Geometry: final body of the model. Coordinates: model frame, mm. A direction names the side the tool comes from. Give positions to 0.01 mm unless a question says otherwise; leave off trailing zeros. Loops run counter-clockwise (first coordinate to the right, second up) from the corner with the lowest first, then second, coordinate; pieces in that order, holes last. Notation, with made-up numbers: (12, 56) -> (69, 56) arc R30 ccw to (69, 82) -> close; hole circle Ø5 at (-33.5, 79.5). An arc over 180 degrees is marked (long way). Answer in a Markdown table with one row per item. Add a question column.
1) Section query C-C (y = 77). Return the cut outline in (x, z), plus the area to 3 significant figures.
2) Section query B-B (x = -15.5). Return the cut outline in (y, z), plus the area to 3 significant figures.
3) Section query D-D (x = 0). Return the cut outline in (y, z), plus the area to 3 significant figures.
4) First-contact query: P1, Ø5, axis at x = -22, z = 4.5, coming from the -Y side; P2, Ø8, axis at x = 16.5, z = 8.5, coming from the -Y side; P3, Ø5, axis at x = 20.5, z = -27, coming from the +Y side. Flat tips, straight axial feed; report the tip coordinate or a pass-through.
5) Section query A-A (z = 0). Return the cut outline in (x, y), plus the area to 3 significant figures.
6) Draft query along Y for faces 1 (the flat face through (-20, -40, 0)), 2 (the flat face through (-8, 0, -1)), 3 (the cylindrical face through (0.33, -9.844, 7.493)), 4 (the flat face through (-8, 5, -1)). Return one class per face: +Y half, -Y half, draft (parallel to the pull), parting line (faces both ways), or undercut.
7) Access query for faces 5 (the cylindrical face through (1.802, 69.09, 5.723)), 6 (the cylindrical face through (-0.28, -28.27, 0.65)), 7 (the flat face through (20, -40, 0)). Directions: +Z, -Z, +X, -X, +Y, -Y. A direction counts if a zero-diameter tool reaches every point of the face in a straight line with its end or side. Return the directions, or none.
8) Line query: line 1 (Y direction, x = 0, z = 0); line 2 (Y direction, x = -26, z = -5); line 3 (Z direction, x = -1, y = 4). Output: solid intervals per line, ascending. Write a range as from..to.
```python
from build123d import *

# Parameters (mm, degrees)
SKETCH4_R           = 39
BOSS_EXTRUDE2_DEPTH = 5
SKETCH5_R           = 6
BOSS_EXTRUDE3_DEPTH = 130
SKETCH6_R           = 7.5
BOSS_EXTRUDE4_DEPTH = 20
SKETCH8_R           = 15.233231967
SKETCH8_R_2         = 5
BOSS_EXTRUDE5_DEPTH = 20


with BuildPart() as part:
    # Sketch4 → Boss-Extrude2 (new body)
    with BuildSketch(Plane(origin=(0, 0, 0), x_dir=(1, 0, 0), z_dir=(0, 1, 0))):
        with Locations(Location((0, 0, 0), (0, 0, 270))):
            Circle(SKETCH4_R)
    extrude(amount=BOSS_EXTRUDE2_DEPTH)

    # Sketch5 → Boss-Extrude3 (add)
    with BuildSketch(Plane(origin=(0, 5, 0), x_dir=(1, 0, 0), z_dir=(0, 1, 0))):
        with Locations(Location((0, 0, 0), (0, 0, 270))):
            Circle(SKETCH5_R)
    extrude(amount=BOSS_EXTRUDE3_DEPTH)

    # Sketch6 → Boss-Extrude4 (add)
    with BuildSketch(Plane.XZ):
        with Locations(Location((0, 0, 0), (0, 0, 270))):
            Circle(SKETCH6_R)
    extrude(amount=BOSS_EXTRUDE4_DEPTH)

    # Sketch8 → Boss-Extrude5 (add, symmetric)
    with BuildSketch(Plane(origin=(0, 0, 0), x_dir=(0, 0, -1), z_dir=(1, 0, 0))):
        with Locations((0, -33.226479946)):
            Circle(SKETCH8_R)
        with Locations((0, -33.226479946)):
            Circle(SKETCH8_R_2, mode=Mode.SUBTRACT)
    extrude(amount=BOSS_EXTRUDE5_DEPTH, both=True)


solid = part.part
```
Evaluation:
| question | item | result |
|---|---|---|
| 1 | outline | circle Ø12 at (0, 0) |
| 1 | area | 113 mm² |
| 2 | outline | circle Ø30.47 at (-33.23, 0); (0, -35.79) -> (5, -35.79) -> (5, 35.79) -> (0, 35.79) -> close; hole circle Ø10 at (-33.23, 0) |
| 2 | area | 1,010 mm² |
| 3 | outline | (-19.97, -7.5) -> (0, -7.5) -> (0, -39) -> (5, -39) -> (5, -6) -> (135, -6) -> (135, 6) -> (5, 6) -> (5, 39) -> (0, 39) -> (0, 7.5) -> (-19.97, 7.5) arc R15.23 ccw (long way) to start; hole circle Ø10 at (-33.23, 0) |
| 3 | area | 2,880 mm² |
| 4 | P1 | y = -48.16 |
| 4 | P2 | y = -47.78 |
| 4 | P3 | y = 5 |
| 5 | outline | (-39, 0) -> (-7.5, 0) -> (-7.5, -17.99) -> (-20, -17.99) -> (-20, -28.23) -> (20, -28.23) -> (20, -17.99) -> (7.5, -17.99) -> (7.5, 0) -> (39, 0) -> (39, 5) -> (6, 5) -> (6, 135) -> (-6, 135) -> (-6, 5) -> (-39, 5) -> close; (-20, -48.46) -> (20, -48.46) -> (20, -38.23) -> (-20, -38.23) -> close |
| 5 | area | 3,040 mm² |
| 6 | face 1 | draft |
| 6 | face 2 | undercut |
| 6 | face 3 | undercut |
| 6 | face 4 | +Y half |
| 7 | face 5 | +Y |
| 7 | face 6 | +X, -X |
| 7 | face 7 | +Z, -Z, +X, -Y |
| 8 | line 1 | -48.46..-38.23, -28.23..135 |
| 8 | line 2 | 0..5 |
| 8 | line 3 | -38.99..38.99 |
